Input: part model. Units: mm. Frame: model coordinates. Coordinates: 2 decimals unless noted, no trailing zeros. Loops run counter-clockwise (first coordinate to the right, second up) from the corner with the lowest first, then second, coordinate; pieces in that order, holes last. Notation, with made-up numbers: (64.25, 3.5) -> (69.25, 3.5) arc R9 cw to (69.25, 19.5) -> close; hole circle Ø1 at (25.5, 79). An arc over 180 degrees is marked (long way). Put each result on its own line as item: value. Start each with the question number.
1) Material intervals for L1, parallel to Y at x = -0.3, z = 73; L2, parallel to Z at x = -0.65, y = 24.75; L3, parallel to Y at x = 0.25, z = 230, sorted ascending.
2) Cut plane C-C (x = -0.2). State how many separate pieces and enclosed holes the cut face has, plus the area to 3 significant figures.
3) Cut plane B-B (z = 73). Return the cut outline in (x, y).
4) Cut plane A-A (z = 230). Return the cut outline in (x, y).
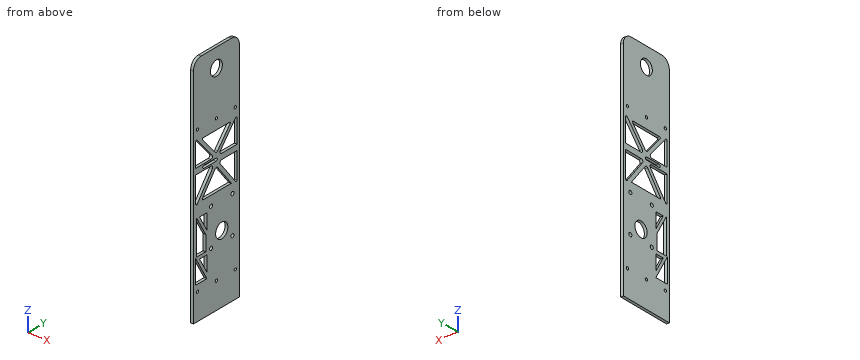
from build123d import *

# Parameters (mm, degrees)
SKETCH1_W           = 3
SKETCH1_H           = 60
BOSS_EXTRUDE1_DEPTH = 250
FILLET1_R           = 10
FILLET2_R           = 10
SKETCH2_R           = 4.25
CUT_EXTRUDE1_DEPTH  = 4
SKETCH5_R           = 7.8
CUT_EXTRUDE4_DEPTH  = 4
SKETCH13_R          = 7.98
CUT_EXTRUDE10_DEPTH = 4
SKETCH14_R          = 2
CUT_EXTRUDE11_DEPTH = 4
CUT_EXTRUDE14_DEPTH = 10
FILLET3_R           = 1
FILLET4_R           = 2
CUT_EXTRUDE18_DEPTH = 10
CUT_EXTRUDE19_DEPTH = 4
SKETCH20_R          = 1.499999993
SKETCH20_R_2        = 1.5
CUT_EXTRUDE20_DEPTH = 4


with BuildPart() as part:
    # Sketch1 → Boss-Extrude1 (new body)
    with BuildSketch(Plane.XY):
        Rectangle(SKETCH1_W, SKETCH1_H)
    extrude(amount=BOSS_EXTRUDE1_DEPTH)

    # Fillet1
    fillet1_edges = [part.edges().sort_by_distance(p)[0] for p in [
        (0, 30, 250),
    ]]
    fillet(fillet1_edges, radius=FILLET1_R)

    # Fillet2
    fillet2_edges = [part.edges().sort_by_distance(p)[0] for p in [
        (0, -30, 250),
    ]]
    fillet(fillet2_edges, radius=FILLET2_R)

    # Sketch2 → Cut-Extrude1 (cut, through all)
    with BuildSketch(Plane.ZY.offset(1.5)):
        with Locations((230, 0)):
            Circle(SKETCH2_R)
    extrude(amount=-CUT_EXTRUDE1_DEPTH, mode=Mode.SUBTRACT)

    # Sketch5 → Cut-Extrude4 (cut, through all)
    with BuildSketch(Plane.ZY.offset(1.5)):
        with Locations((230, 0)):
            Circle(SKETCH5_R)
    extrude(amount=-CUT_EXTRUDE4_DEPTH, mode=Mode.SUBTRACT)

    # Sketch13 → Cut-Extrude10 (cut, through all)
    with BuildSketch(Plane.ZY.offset(1.5)):
        with Locations((73, 7)):
            Circle(SKETCH13_R)
    extrude(amount=-CUT_EXTRUDE10_DEPTH, mode=Mode.SUBTRACT)

    # Sketch14 → Cut-Extrude11 (cut, through all)
    with BuildSketch(Plane(origin=(1.5, 0, 0), x_dir=(0, 0, -1), z_dir=(1, 0, 0))):
        with Locations((-102, -7)):
            Circle(SKETCH14_R)
        with Locations((-102, 21)):
            Circle(SKETCH14_R)
        with Locations((-62, 21)):
            Circle(SKETCH14_R)
        with Locations((-62, -7)):
            Circle(SKETCH14_R)
    extrude(amount=-CUT_EXTRUDE11_DEPTH, mode=Mode.SUBTRACT)

    # Sketch17 → Cut-Extrude14 (cut)
    with BuildSketch(Plane.ZY.offset(1.5)):
        Polygon((149.1019184, 0), (171.275987572, -19.368578167), (171.275987572, 19.368578167), align=None)
        Polygon((146.3902575, -27), (174.288564399, -27), (146.3902575, -2.631421833), align=None)
        Polygon((109.288564399, -27), (140.055353087, -27), (140.055353087, -2.631421833), align=None)
        Polygon((112.424175394, 19.516465485), (112.424175394, -19.516465485), (137.064881363, 0), align=None)
        Polygon((109.288564399, 27), (140.242069678, 2.483534515), (140.242069678, 27), align=None)
        Polygon((146.220949067, 2.483534515), (174.288564399, 27), (146.220949067, 27), align=None)
    extrude(amount=-CUT_EXTRUDE14_DEPTH, mode=Mode.SUBTRACT)

    # Fillet3
    fillet3_edges = [part.edges().sort_by_distance(p)[0] for p in [
        (0, -27, 174.288564399),
        (0, 27, 174.288564399),
        (0, -19.368578167, 171.275987572),
        (0, 19.368578167, 171.275987572),
        (0, -19.516465485, 112.424175394),
        (0, 27, 109.288564399),
        (0, -27, 109.288564399),
    ]]
    fillet(fillet3_edges, radius=FILLET3_R)

    # Fillet4
    fillet4_edges = [part.edges().sort_by_distance(p)[0] for p in [
        (0, -2.631421833, 146.3902575),
        (0, 2.483534515, 146.220949067),
        (0, 0, 149.1019184),
        (0, 0, 137.064881363),
        (0, 2.483534515, 140.242069678),
        (0, -2.631421833, 140.055353087),
    ]]
    fillet(fillet4_edges, radius=FILLET4_R)

    # Sketch18 → Cut-Extrude18 (cut)
    with BuildSketch(Plane.ZY.offset(1.5)):
        Polygon((61.668054604, -26), (98.988380185, -26), (78.023904982, -13.896154598), (61.668054604, -13.896154598), align=None)
        Polygon((98.086456396, -21.955043464), (98.086456396, -12.396154598), (81.529975217, -12.396154598), align=None)
        Polygon((58.14382401, -12.396154598), (41.612161756, -12.396154598), (58.14382401, -21.940994237), align=None)
        Polygon((35.508194368, -27.5), (61.668054604, -27.5), (35.508194368, -12.396154598), align=None)
    extrude(amount=-CUT_EXTRUDE18_DEPTH, mode=Mode.SUBTRACT)

    # Sketch19 → Cut-Extrude19 (cut, through all)
    with BuildSketch(Plane.ZY.offset(1.5)):
        with BuildLine():
            Line((144.8152575, -0.290513908), (144.8152575, -16.383557477))
            ThreePointArc((144.8152575, -16.383557477), (143.3152575, -17.883557477), (141.8152575, -16.383557477))
            Line((141.8152575, -16.383557477), (141.8152575, -0.290513908))
            ThreePointArc((141.8152575, -0.290513908), (143.3152575, 1.209486092), (144.8152575, -0.290513908))
        make_face()
    extrude(amount=-CUT_EXTRUDE19_DEPTH, mode=Mode.SUBTRACT)

    # Sketch20 → Cut-Extrude20 (cut, through all)
    with BuildSketch(Plane.ZY.offset(1.5)):
        with Locations((28.351822222, -24.750000002)):
            Circle(SKETCH20_R)
        with Locations((28.351822222, -2e-09)):
            Circle(SKETCH20_R)
        with Locations((28.351822222, 24.749999998)):
            Circle(SKETCH20_R)
        with Locations((182.288564399, -24.750000007)):
            Circle(SKETCH20_R_2)
        with Locations((182.288564399, -7e-09)):
            Circle(SKETCH20_R_2)
        with Locations((182.288564399, 24.749999993)):
            Circle(SKETCH20_R_2)
    extrude(amount=-CUT_EXTRUDE20_DEPTH, mode=Mode.SUBTRACT)


solid = part.part
Results found:
1. L1: y = -30 to -26, -13.9 to -0.98, 14.98 to 30
1. L2: z = 0 to 26.85, 29.85 to 112.13, 140.24 to 146.22, 171.71 to 180.79, 183.79 to 248.8
1. L3: y = -30 to -7.8, 7.8 to 30
2. separate pieces: 1
2. enclosed holes: 23
2. area: 11,400 mm2
3. outline: (-1.5, -30) -> (1.5, -30) -> (1.5, -26) -> (-1.5, -26) -> close; (-1.5, -13.9) -> (1.5, -13.9) -> (1.5, -0.98) -> (-1.5, -0.98) -> close; (-1.5, 14.98) -> (1.5, 14.98) -> (1.5, 30) -> (-1.5, 30) -> close
4. outline: (-1.5, -30) -> (1.5, -30) -> (1.5, -7.8) -> (-1.5, -7.8) -> close; (-1.5, 7.8) -> (1.5, 7.8) -> (1.5, 30) -> (-1.5, 30) -> close
